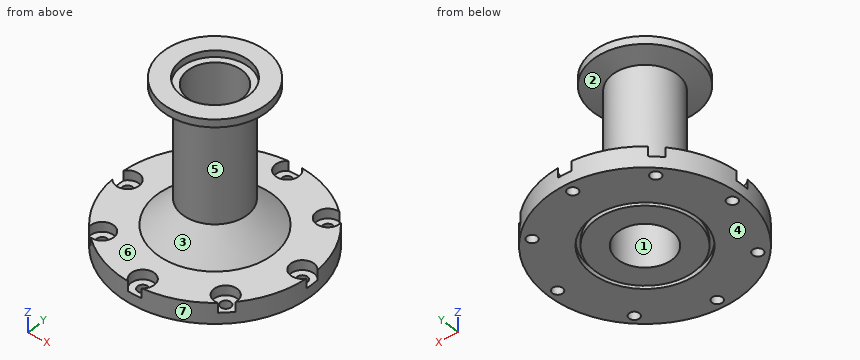
from build123d import *

# Parameters (mm, degrees)
SKETCH2_R           = 37.5
SKETCH2_R_2         = 5.35
BOSS_EXTRUDE2_DEPTH = 8
SKETCH14_R          = 2
CUT_EXTRUDE6_DEPTH  = 54.633012222
SKETCH3_R           = 20.71
SKETCH3_R_2         = 19.21
CUT_EXTRUDE2_DEPTH  = 2
SKETCH7_R           = 12.5
SKETCH7_R_2         = 10.5
BOSS_EXTRUDE4_DEPTH = 50.8
SKETCH10_R          = 12.5
BOSS_EXTRUDE5_DEPTH = 2.01
BOSS_EXTRUDE5_DRAFT = -75
SKETCH11_R          = 10.5
CUT_EXTRUDE3_DEPTH  = 81.686777727
BOSS_EXTRUDE6_START = 3
SKETCH12_R          = 20.001422123
SKETCH12_R_2        = 10.5
BOSS_EXTRUDE6_DEPTH = 3
SKETCH13_R          = 13.1
CUT_EXTRUDE4_DEPTH  = 2.5
CHAMFER1_SIZE       = 10
SKETCH17_R          = 4.5
CUT_EXTRUDE8_DEPTH  = 3.75


with BuildPart() as part:
    # Sketch2 → Boss-Extrude2 (new body)
    with BuildSketch(Plane.XY):
        Circle(SKETCH2_R)
        Circle(SKETCH2_R_2, mode=Mode.SUBTRACT)
    extrude(amount=BOSS_EXTRUDE2_DEPTH)

    # Sketch14 → Cut-Extrude6 (cut, through all)
    with BuildSketch(Plane.XY):
        with Locations((0, 33.75)):
            Circle(SKETCH14_R)
        with Locations((-23.864853865, 23.864853865)):
            Circle(SKETCH14_R)
        with Locations((-33.75, 0)):
            Circle(SKETCH14_R)
        with Locations((-23.864853865, -23.864853865)):
            Circle(SKETCH14_R)
        with Locations((0, -33.75)):
            Circle(SKETCH14_R)
        with Locations((23.864853865, -23.864853865)):
            Circle(SKETCH14_R)
        with Locations((33.75, 0)):
            Circle(SKETCH14_R)
        with Locations((23.864853865, 23.864853865)):
            Circle(SKETCH14_R)
    extrude(amount=CUT_EXTRUDE6_DEPTH, mode=Mode.SUBTRACT)

    # Sketch3 → Cut-Extrude2 (cut)
    with BuildSketch(Plane.XY):
        Circle(SKETCH3_R)
        Circle(SKETCH3_R_2, mode=Mode.SUBTRACT)
    extrude(amount=CUT_EXTRUDE2_DEPTH, mode=Mode.SUBTRACT)

    # Sketch7 → Boss-Extrude4 (add)
    with BuildSketch(Plane.XY.offset(8)):
        Circle(SKETCH7_R)
        Circle(SKETCH7_R_2, mode=Mode.SUBTRACT)
    extrude(amount=BOSS_EXTRUDE4_DEPTH)


with BuildPart() as boss_extrude5_tool:
    # Sketch10 → Boss-Extrude5 (with draft: the straight prism first)
    with BuildSketch(Plane.XY.offset(58.8)):
        Circle(SKETCH10_R)
    extrude(amount=BOSS_EXTRUDE5_DEPTH)
    # Boss-Extrude5: the draft: its side faces are tilted about the plane it starts from
    boss_extrude5_sides = [boss_extrude5_tool.faces().sort_by_distance(p)[0] for p in [
        (-12.5, 0, 59.805),
    ]]
    draft(boss_extrude5_sides, Plane.XY.offset(58.8), BOSS_EXTRUDE5_DRAFT)


with BuildPart() as part_1:
    add(part.part)

    # Boss-Extrude5: add boss_extrude5_tool
    add(boss_extrude5_tool.part)

    # Sketch11 → Cut-Extrude3 (cut, through all)
    with BuildSketch(Plane.XY.offset(60.81)):
        Circle(SKETCH11_R)
    extrude(amount=-CUT_EXTRUDE3_DEPTH, mode=Mode.SUBTRACT)

    # Sketch12 → Boss-Extrude6 (add)
    with BuildSketch(Plane.XY.offset(60.81).offset(BOSS_EXTRUDE6_START)):
        Circle(SKETCH12_R)
        Circle(SKETCH12_R_2, mode=Mode.SUBTRACT)
    extrude(amount=-BOSS_EXTRUDE6_DEPTH)

    # Sketch13 → Cut-Extrude4 (cut)
    with BuildSketch(Plane.XY.offset(63.81)):
        Circle(SKETCH13_R)
    extrude(amount=-CUT_EXTRUDE4_DEPTH, mode=Mode.SUBTRACT)

    # Chamfer1
    chamfer1_edges = [part_1.edges().sort_by_distance(p)[0] for p in [
        (-12.5, 0, 8),
    ]]
    chamfer(chamfer1_edges, length=CHAMFER1_SIZE)

    # Sketch17 → Cut-Extrude8 (cut)
    with BuildSketch(Plane.XY.offset(8)):
        with Locations((-23.864853865, 23.864853865)):
            Circle(SKETCH17_R)
        with Locations((-33.75, 0)):
            Circle(SKETCH17_R)
        with Locations((0, 33.75)):
            Circle(SKETCH17_R)
        with Locations((23.864853865, 23.864853865)):
            Circle(SKETCH17_R)
        with Locations((33.75, 0)):
            Circle(SKETCH17_R)
        with Locations((23.864853865, -23.864853865)):
            Circle(SKETCH17_R)
        with Locations((0, -33.75)):
            Circle(SKETCH17_R)
        with Locations((-23.864853865, -23.864853865)):
            Circle(SKETCH17_R)
    extrude(amount=-CUT_EXTRUDE8_DEPTH, mode=Mode.SUBTRACT)


solid = part_1.part
Could you check a few things on this model? Use its own coordinates, in mm. Face numbers are marked on the shaded views. A direction names the side the tool comes from. Coordinates: 2 decimals unless noted, no trailing zeros. Loops run counter-clockwise (first coordinate to the right, second up) from the corner with the lowest first, then second, coordinate; pieces in that order, holes last.
1. For the marked faces 5, 6 and 7, which set-ups out of +Z, -Z, +X, -X, +Y, -Y let a thin tool reach every point of the face, with its end or its side?
2. Imagine slicing it at D-D (x = 0). Give the number of separate pieces and of enclosed holes in the cut face, and give its area (3 significant figures).
3. I need wall thicknesses on L1, parallel to Y at x = 0, z = 6; L2, parallel to Z at x = 12, y = 20; L3, parallel to Z at x = 2, y = -12.5. Which ranges of each line are inside material? Lowest first, please.
4. We'd pull the mould along Z, two halves only. Please class the marked faces 1, 2, 3 and 4: released by +Z, released by -Z, zero draft, split by the parting line, or undercut.
5. Imagine slicing it at C-C (z = 40). Please give me the cut outline in (x, y).
6. For P1, Ø6.5, axis at x = -0.5, y = 35, coming from the +Z side; P2, Ø4.5, axis at x = 22, y = 23, coming from the +Z side; P3, Ø6, axis at x = 13.5, z = 28, coming from the +Y side, each with a flat end and sliding along its axis, tell me the tip position at first contact or that it passes through.
7. Imagine slicing it at A-A (x = 33.75). Please give me the cut outline in (y, z).
Computed values:
1. face 5: none
1. face 6: +Z
1. face 7: +Z, -Z
2. separate pieces: 4
2. enclosed holes: 0
2. area: 700 mm2
3. L1: y = -29.25 to -10.5, 10.5 to 29.25
3. L2: z = 0 to 8
3. L3: z = 0 to 17.84, 58.84 to 61.31
4. face 1: zero draft
4. face 2: undercut
4. face 3: undercut
4. face 4: released by -Z
5. outline: circle Ø25 at (0, 0); hole circle Ø21 at (0, 0)
6. P1: stops at z = 8
6. P2: stops at z = 4.25
6. P3: stops at y = 6.78
7. outline: (-16.35, 0) - (-2, 0) - (-2, 4.25) - (-4.5, 4.25) - (-4.5, 8) - (-16.35, 8) - close; (2, 0) - (16.35, 0) - (16.35, 8) - (4.5, 8) - (4.5, 4.25) - (2, 4.25) - close
